Part print with two shaded views. Sizes in mm from the minimum x, y, z corner. A direction names the side the tool comes from. Round coordinates to 2 decimals unless told otherwise and drop trailing zeros. Write each loop counter-clockwise with the first axis right and the second up, starting at its lowest first coordinate (ties: lowest second). Pieces come first, ordered by that corner, then holes.
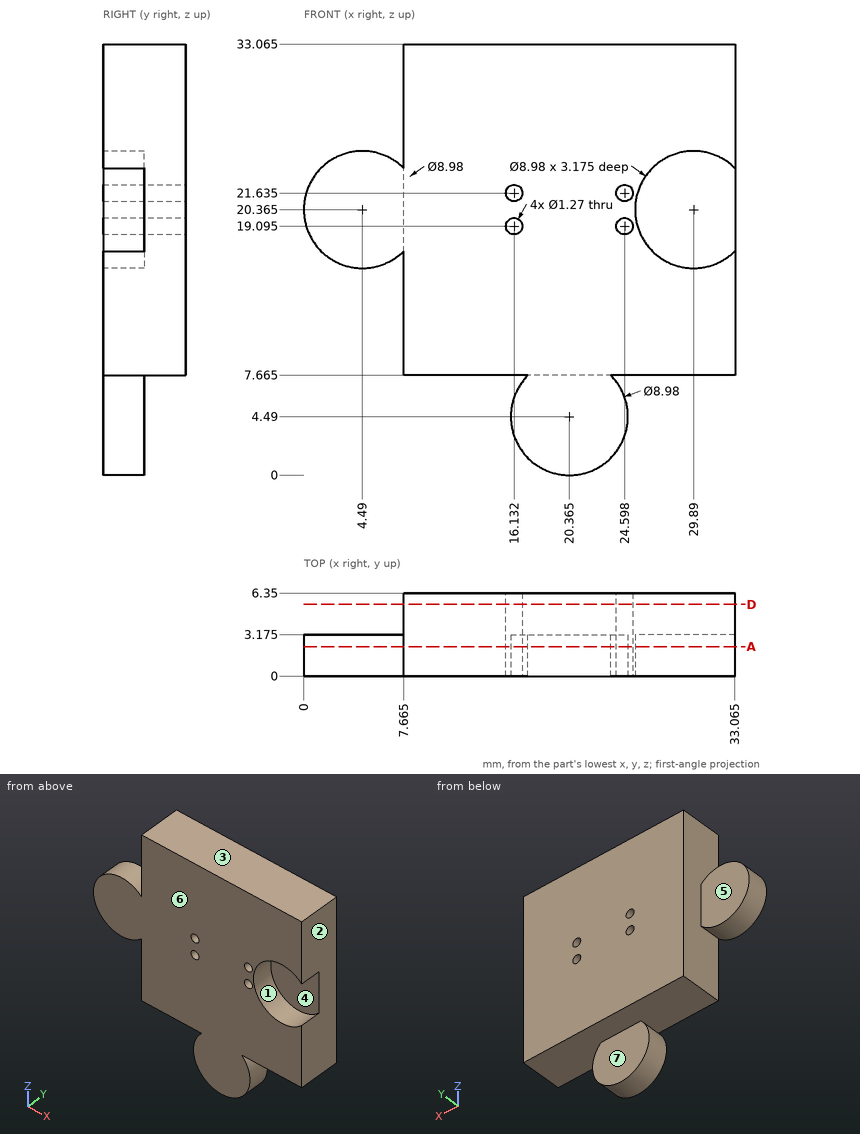
Q1. Cut at D-D on y = 5.5. Write the cut outline in (x, z) (1 decimal), plus the area to 3 significant figures.
Values follow:
outline: (7.7, 7.7) - (33.1, 7.7) - (33.1, 33.1) - (7.7, 33.1) - close; hole circle Ø1.3 at (16.1, 19.1); hole circle Ø1.3 at (16.1, 21.6); hole circle Ø1.3 at (24.6, 19.1); hole circle Ø1.3 at (24.6, 21.6)
area: 640 mm2
Q2. Drop flat-ended pins along their axis: pin 1 (0.8 mm diameter, centred on x = 24.6, z = 19.1, fed in from +Y); pin 2 (4 mm diameter, centred on x = 19, z = 2.5, fed in from +Y) (3 decimals); pin 3 (2 mm diameter, centred on y = 5, z = 16.5, fed in from -X) (1 decimal); pin 4 (4 mm diameter, centred on x = 29, z = 21.5, fed in from -Y) (3 decimals). Give the stop position or say it passes through.
Values follow:
pin 1: passes through
pin 2: stops at y = 3.175
pin 3: stops at x = 7.7
pin 4: stops at y = 3.175
Q3. Mould opens along X. For the marked faces 1, 2 and 3 say: +X half, -X half, draft (parallel to the pull), parting line (faces both ways), or undercut.
Values follow:
face 1: undercut
face 2: +X half
face 3: draft
Q4. Cut at A-A on y = 2.25. Write the cut outline in (x, z) (1 decimal), plus the area to 3 significant figures.
Values follow:
outline: (7.7, 7.7) - (17.2, 7.7) arc R4.5 ccw (long way) to (23.5, 7.7) - (33.1, 7.7) - (33.1, 17.2) arc R4.5 cw (long way) to (33.1, 23.5) - (33.1, 33.1) - (7.7, 33.1) - (7.7, 23.5) arc R4.5 ccw (long way) to (7.7, 17.2) - close; hole circle Ø1.3 at (16.1, 19.1); hole circle Ø1.3 at (16.1, 21.6); hole circle Ø1.3 at (24.6, 19.1); hole circle Ø1.3 at (24.6, 21.6)
area: 698 mm2
Q5. Which spindle directions (+Z, -Z, +X, -X, +Y, -Y) get a long thin tool onto all of the face, cutting with end or side? Do the marked faces 4, 5, 6 and 7. Say none if no direction does.
Values follow:
face 4: -Y
face 5: +Z, -Z, -X, +Y
face 6: +Z, -Z, +X, -X, -Y
face 7: -Z, +X, -X, +Y
Q6. Wall check: L1, parallel to Z at x = 30, y = 1 (1 decimal); L2, parallel to X at y = 2.75, z = 15 (1 decimal); L3, parallel to Z at x = 31.5, y = 1.5 (1 decimal). Give the ranges that are in metal, low to high.
Values follow:
L1: z = 7.7 to 15.9, 24.9 to 33.1
L2: x = 7.7 to 33.1
L3: z = 7.7 to 16.2, 24.6 to 33.1
